Here's the drawing with two shaded views (mm, measured from the low corner). I have some questions. Coordinates: 2 decimals unless noted, no trailing zeros. Write each loop counter-clockwise with the first axis right and the second up, starting at its lowest first coordinate (ties: lowest second). Pieces come first, ordered by that corner, then holes. Notation, with made-up numbers: (39, -25) - (64, -25) arc R24 ccw to (64, 13) - close; hole circle Ø7 at (87, 31.5). An arc over 180 degrees is marked (long way). Answer in a Markdown table with one row per item. Add a question column.
Item 1: Imagine slicing it at A-A (y = 9). Please give me the cut outline in (x, z).
Item 2: Imagine slicing it at C-C (x = 35). Please give me the cut outline in (y, z), plus the area to 3 significant figures.
Item 3: I'm going to push flat-ended pins straight in: pin 1 (1.2 mm diameter, centred on x = 6.5, z = 7.5, fed in from -Y); pin 2 (2 mm diameter, centred on x = 11.5, z = 10, fed in from -Y); pin 3 (5 mm diameter, centred on x = 19, z = 7, fed in from +Y). Where does each tip first touch, or does it pass through?
Item 4: Imagine slicing it at D-D (z = 9.75). State how many separate pieces and enclosed holes the cut face has, plus the area to 3 significant figures.
Item 5: If I drill on probe 1 along X at (y, z) = (30, 12) (1 decimal); probe 2 along Z at (x, y) = (19, 36.5); probe 3 along X at (y, z) = (14, 7.5), over which ranges is the centre line in solid material (lowest first)? Write a range as from..to.
Item 6: We'd pull the mould along X, two halves only. Please class the marked faces 1, 2, 3 and 4: +X half, -X half, draft (parallel to the pull), parting line (faces both ways), or undercut.
Item 7: Imagine slicing it at B-B (y = 34.5). Please give me the cut outline in (x, z), plus the area to 3 significant figures.
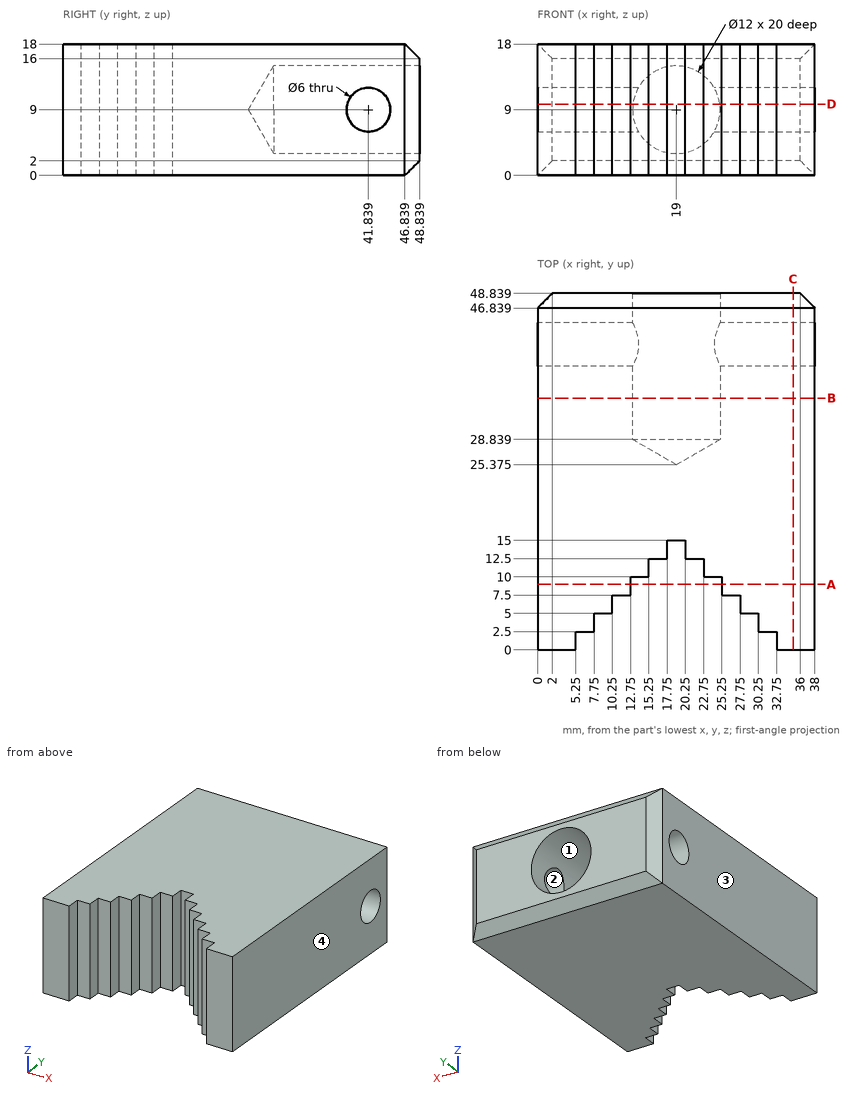
Here are the results:
| question | item | result |
|---|---|---|
| 1 | outline | (0, 0) - (12.75, 0) - (12.75, 18) - (0, 18) - close; (25.25, 0) - (38, 0) - (38, 18) - (25.25, 18) - close |
| 2 | outline | (0, 0) - (46.84, 0) - (48.84, 2) - (48.84, 16) - (46.84, 18) - (0, 18) - close; hole circle Ø6 at (41.84, 9) |
| 2 | area | 847 mm2 |
| 3 | pin 1 | stops at y = 2.5 |
| 3 | pin 2 | stops at y = 7.5 |
| 3 | pin 3 | stops at y = 27.97 |
| 4 | separate pieces | 3 |
| 4 | enclosed holes | 0 |
| 4 | area | 1,220 mm2 |
| 5 | probe 1 | x = 0..13.8, 24.2..38 |
| 5 | probe 2 | z = 0..3, 15..18 |
| 5 | probe 3 | x = 0..17.75, 20.25..38 |
| 6 | face 1 | undercut |
| 6 | face 2 | draft |
| 6 | face 3 | -X half |
| 6 | face 4 | +X half |
| 7 | outline | (0, 0) - (38, 0) - (38, 18) - (0, 18) - close; hole circle Ø12 at (19, 9) |
| 7 | area | 571 mm2 |
